Here's how the part is built. I have some questions about the finished solid (model axes, mm). A direction names the side the tool comes from. Round coordinates to 2 decimals unless told otherwise and drop trailing zeros. Order: outer loops, then holes, each group sorted by start corner. A loop starts at its lowest first (then second) coordinate and runs counter-clockwise, first axis right, second up. Notation, with made-up numbers: (-27, 78.25) - (8, 78.25) arc R8 cw to (8, 93.25) - close; hole circle Ø6 at (75, -35.75). An arc over 180 degrees is marked (long way). Answer as a JSON object with one key per item and string values.
```python
from build123d import *

# Parameters (mm, degrees)
F0_W     = 401
F0_H     = 171
F0_R     = 3
F0_R_2   = 3.627457
F0_W_2   = 121
F0_H_2   = 121
F1_DEPTH = 10
F2_R     = 5


with BuildPart() as f1:
    # F0 (on Top) → F1 (new body)
    with BuildSketch(Plane.XY):
        with Locations((60.5, -60.5)):
            Rectangle(F0_W, F0_H)
        with Locations((-127, -135.5)):
            Circle(F0_R, mode=Mode.SUBTRACT)
        with Locations((248, -135.5)):
            Circle(F0_R_2, mode=Mode.SUBTRACT)
        with Locations((-65.5, -60.5)):
            Rectangle(F0_W_2, F0_H_2, mode=Mode.SUBTRACT)
        with Locations((-127, 14.5)):
            Circle(F0_R, mode=Mode.SUBTRACT)
        with Locations((60.5, -60.5)):
            Rectangle(F0_W_2, F0_H_2, mode=Mode.SUBTRACT)
        with Locations((186.5, -60.5)):
            Rectangle(F0_W_2, F0_H_2, mode=Mode.SUBTRACT)
        with Locations((248, 14.5)):
            Circle(F0_R_2, mode=Mode.SUBTRACT)
    extrude(amount=F1_DEPTH)

    # F2
    f2_edges = [f1.edges().sort_by_distance(p)[0] for p in [
        (261, 25, 5),
        (261, -146, 5),
        (-140, -146, 5),
        (-140, 25, 5),
    ]]
    fillet(f2_edges, radius=F2_R)


solid = f1.part
```
1. Imagine slicing it at C-C (x = 193). List the corners of the cut face in (y, z) for me.
Responses:
{"outline": "(-146, 0) - (-121, 0) - (-121, 10) - (-146, 10) - close; (0, 0) - (25, 0) - (25, 10) - (0, 10) - close"}
2. Imagine slicing it at B-B (z = 2.75). List the corners of the cut face in (x, y) for me.
Responses:
{"outline": "(-140, -141) arc R5 ccw to (-135, -146) - (256, -146) arc R5 ccw to (261, -141) - (261, 20) arc R5 ccw to (256, 25) - (-135, 25) arc R5 ccw to (-140, 20) - close; hole circle Ø6 at (-127, -135.5); hole circle Ø6 at (-127, 14.5); hole (-126, -121) - (-5, -121) - (-5, 0) - (-126, 0) - close; hole (0, -121) - (121, -121) - (121, 0) - (0, 0) - close; hole (126, -121) - (247, -121) - (247, 0) - (126, 0) - close; hole circle Ø7.25 at (248, -135.5); hole circle Ø7.25 at (248, 14.5)"}
3. For faces 4 (the face through (-126, -61, 5)), 5 (the face through (58, -146, 5)), which set-ups out of +Z, -Z, +X, -X, +Y, -Y let a thin tool reach every point of the face, with its end or its side?
Responses:
{"face 4": "+Z, -Z", "face 5": "+Z, -Z, +X, -X, -Y"}
4. Thinking about a two-plate mould opening in X: for faces 1 (the face through (186, 0, 5)), 2 (the face through (60, 3, 10)), 3 (the face through (-140, -62, 5)), which applies, pulls with the +X half, pulls with the -X half, needs draft (parallel to the pull), parting line crosses it, or undercut?
Responses:
{"face 1": "undercut", "face 2": "needs draft", "face 3": "pulls with the -X half"}
5. If I drill on L1, parallel to Y at x = 248, z = 7.5; L2, parallel to X at y = -108, z = 9.5; L3, parallel to X at y = -135.5, z = 7.75, over which ranges is the centre line in solid material (lowest first)? Write a range as [from, to].
Responses:
{"L1": "[-146, -139.13], [-131.87, 10.87], [18.13, 25]", "L2": "[-140, -126], [-5, 0], [121, 126], [247, 261]", "L3": "[-140, -130], [-124, 244.37], [251.63, 261]"}
6. Imagine slicing it at A-A (y = -116). List the corners of the cut face in (x, z) for me.
Responses:
{"outline": "(-140, 0) - (-126, 0) - (-126, 10) - (-140, 10) - close; (-5, 0) - (0, 0) - (0, 10) - (-5, 10) - close; (121, 0) - (126, 0) - (126, 10) - (121, 10) - close; (247, 0) - (261, 0) - (261, 10) - (247, 10) - close"}
